from build123d import *

# Parameters (mm, degrees)
ESBO_O2_W                = 200
ESBO_O2_H                = 100
RESSALTO_EXTRUS_O1_DEPTH = 50
FILETE1_R                = 50
ESBO_O3_R                = 15
CORTE_EXTRUS_O1_DEPTH    = 25
ESBO_O4_R                = 10
CORTE_EXTRUS_O2_DEPTH    = 123.474487139


with BuildPart() as part:
    # Esboço2 → Ressalto-extrusão1 (new body)
    with BuildSketch(Plane(origin=(0, 0, 0), x_dir=(1, 0, 0), z_dir=(0, 1, 0))):
        Rectangle(ESBO_O2_W, ESBO_O2_H)
    extrude(amount=RESSALTO_EXTRUS_O1_DEPTH)

    # Filete1
    filete1_edges = [part.edges().sort_by_distance(p)[0] for p in [
        (100, 25, -50),
        (100, 25, 50),
        (-100, 25, -50),
        (-100, 25, 50),
    ]]
    fillet(filete1_edges, radius=FILETE1_R - 0.0001)  # a hair under: the kernel refuses the full size

    # Esboço3 → Corte-extrusão1 (cut)
    with BuildSketch(Plane.XZ):
        with Locations(Location((50, 0, 0), (0, 0, 270))):
            Circle(ESBO_O3_R)
    extrude(amount=-CORTE_EXTRUS_O1_DEPTH, mode=Mode.SUBTRACT)

    # Esboço4 → Corte-extrusão2 (cut, through all)
    with BuildSketch(Plane.XZ):
        with Locations(Location((-50, 0, 0), (0, 0, 270))):
            Circle(ESBO_O4_R)
    extrude(amount=-CORTE_EXTRUS_O2_DEPTH, mode=Mode.SUBTRACT)


solid = part.part
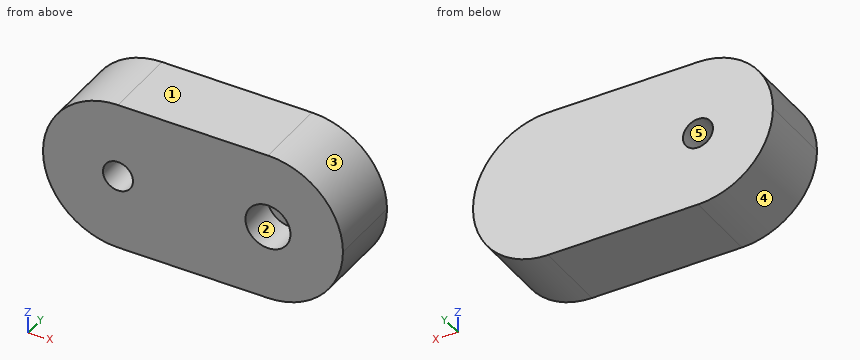
Model file for the job. Use its own axes, mm. Face numbers are marked on the shaded views. A direction names the side the tool comes from. Give positions to 0.01 mm unless a question says otherwise; leave off trailing zeros. Loops run counter-clockwise (first coordinate to the right, second up) from the corner with the lowest first, then second, coordinate; pieces in that order, holes last.
Item 1: Slice it at A-A (y = 18). Give the number of separate pieces and of enclosed holes in the cut face, plus the area to 3 significant figures.
Check values:
separate pieces: 1
enclosed holes: 2
area: 16,800 mm2
Item 2: Mould opens along Z. For the marked faces 3, 4 and 5 say: +Z half, -Z half, draft (parallel to the pull), parting line (faces both ways), or undercut.
Check values:
face 3: +Z half
face 4: -Z half
face 5: undercut
Item 3: Drill centre lines: line 1 along X through (y, z) = (19, 0); line 2 along X through (y, z) = (21, -9); line 3 along Z through (x, y) = (-43.5, 20). Where is each one in solid material? Low to high.
Check values:
line 1: x = -100 to -60, -40 to 35, 65 to 100
line 2: x = -99.18 to -54.36, -45.64 to 38, 62 to 99.18
line 3: z = -50 to -7.6, 7.6 to 50
Item 4: Slice it at D-D (x = 48). Write the cut outline in (y, z), plus the area to 3 significant figures.
Check values:
outline: (0, -50) - (50, -50) - (50, 50) - (0, 50) - (0, 14.87) - (25, 14.87) - (25, -14.87) - (0, -14.87) - close
area: 4,260 mm2
Item 5: Slice it at B-B (x = -57). Write the cut outline in (y, z).
Check values:
outline: (0, -49.51) - (50, -49.51) - (50, -7.14) - (0, -7.14) - close; (0, 7.14) - (50, 7.14) - (50, 49.51) - (0, 49.51) - close
Item 6: Drop flat-ended pins along their axis: P1, Ø10, axis at y = 18, z = -26, coming from the +X side; P2, Ø10, axis at y = 41.5, z = -31.5, coming from the -X side; P3, Ø1, axis at y = 20, z = -19, coming from the +X side; P4, Ø24, axis at x = 43, z = -1, coming from the -Y side. Give the stop position or say it passes through.
Check values:
P1: stops at x = 95.38
P2: stops at x = -92.4
P3: stops at x = 96.45
P4: stops at y = 0
Item 7: Which spindle directions (+Z, -Z, +X, -X, +Y, -Y) get a long thin tool onto all of the face, cutting with end or side? Do the marked faces 1 and 2. Say none if no direction does.
Check values:
face 1: +Z, +X, -X, +Y, -Y
face 2: -Y
